```python
from build123d import *

# Parameters (mm, degrees)
BOSS_EXTRUDE1_DEPTH     = 5
SKETCH2_R               = 1.5
CUT_EXTRUDE1_DEPTH      = 5
CIRPATTERN1_COUNT       = 4
CIRPATTERN1_ANGLE       = 168
SKETCH9_W               = 120
SKETCH9_H               = 25
BOSS_EXTRUDE5_DEPTH     = 5
MIRROR3_COPY_1_SKETCH_R = 1.5
MIRROR3_COPY_1_DEPTH    = 5
MIRROR3_COPY_2_SKETCH_R = 1.5
MIRROR3_COPY_2_DEPTH    = 5
MIRROR3_COPY_3_SKETCH_R = 1.5
MIRROR3_COPY_3_DEPTH    = 5
SKETCH11_W              = 83.519878
SKETCH11_H              = 28.939674
CUT_EXTRUDE2_DEPTH      = 150
CHAMFER1_SIZE           = 1


with BuildPart() as part:
    # Sketch1 → Boss-Extrude1 (new body)
    with BuildSketch(Plane(origin=(0, 0, 0), x_dir=(1, 0, 0), z_dir=(0, 1, 0))):
        with BuildLine():
            Line((-60, 0), (-25.75, 0))
            Line((-25.75, 0), (25.75, 0))
            Line((25.75, 0), (60, 0))
            ThreePointArc((60, 0), (0, 60), (-60, 0))
        make_face()
    boss_extrude1 = extrude(amount=BOSS_EXTRUDE1_DEPTH)

    # Sketch2 → Cut-Extrude1 (cut)
    with BuildSketch(Plane(origin=(0, 5, 0), x_dir=(1, 0, 0), z_dir=(0, 1, 0))):
        with Locations((-54.772256, 5)):
            Circle(SKETCH2_R)
    cut_extrude1 = extrude(amount=-CUT_EXTRUDE1_DEPTH, mode=Mode.SUBTRACT)

    # CirPattern1: Cut-Extrude1 ×4 about axis
    cirpattern1_axis = Axis((0, 0, 0), (0, -1, 0))
    for i in range(1, CIRPATTERN1_COUNT):
        add(cut_extrude1.rotate(cirpattern1_axis, i * CIRPATTERN1_ANGLE / (CIRPATTERN1_COUNT - 1)), mode=Mode.SUBTRACT)

    # Sketch9 → Boss-Extrude5 (add)
    with BuildSketch(Plane.XY):
        with Locations((0, -7.5)):
            Rectangle(SKETCH9_W, SKETCH9_H)
    boss_extrude5 = extrude(amount=BOSS_EXTRUDE5_DEPTH)

    # Mirror3: Boss-Extrude1, Cut-Extrude1, Boss-Extrude5 across plane
    add(boss_extrude1.mirror(Plane.ZX.offset(5)))
    add(cut_extrude1.mirror(Plane.ZX.offset(5)), mode=Mode.SUBTRACT)
    add(boss_extrude5.mirror(Plane.ZX.offset(5)))

    # Mirror3 copy 1 sketch → Mirror3 copy 1 (cut)
    with BuildSketch(Plane(origin=(0, 5, 0), x_dir=(0.559193, 0, 0.829038), z_dir=(0, -1, 0))):
        with Locations((-54.772256, -5)):
            Circle(MIRROR3_COPY_1_SKETCH_R)
    extrude(amount=-MIRROR3_COPY_1_DEPTH, mode=Mode.SUBTRACT)

    # Mirror3 copy 2 sketch → Mirror3 copy 2 (cut)
    with BuildSketch(Plane(origin=(0, 5, 0), x_dir=(-0.374607, 0, 0.927184), z_dir=(0, -1, 0))):
        with Locations((-54.772256, -5)):
            Circle(MIRROR3_COPY_2_SKETCH_R)
    extrude(amount=-MIRROR3_COPY_2_DEPTH, mode=Mode.SUBTRACT)

    # Mirror3 copy 3 sketch → Mirror3 copy 3 (cut)
    with BuildSketch(Plane(origin=(0, 5, 0), x_dir=(-0.978148, 0, 0.207912), z_dir=(0, -1, 0))):
        with Locations((-54.772256, -5)):
            Circle(MIRROR3_COPY_3_SKETCH_R)
    extrude(amount=-MIRROR3_COPY_3_DEPTH, mode=Mode.SUBTRACT)

    # Sketch11 → Cut-Extrude2 (cut)
    with BuildSketch(Plane.ZY.offset(60)):
        with Locations((-36.759939, -9.469837)):
            Rectangle(SKETCH11_W, SKETCH11_H)
    extrude(amount=-CUT_EXTRUDE2_DEPTH, mode=Mode.SUBTRACT)

    # Chamfer1
    chamfer1_edges = [part.edges().sort_by_distance(p)[0] for p in [
        (0, 5, 5),
        (56.08213, 5, -6.808922),
        (-27.321858, 5, -49.447779),
        (60, 5, 2.5),
        (0, 5, -60),
        (25.715877, 5, -50.301694),
        (-56.272256, 5, -5),
        (-60, 5, 2.5),
    ]]
    chamfer(chamfer1_edges, length=CHAMFER1_SIZE)


solid = part.part
```
Source: CAD feature listing. Evaluate the final solid. Frame: model axes, mm. A direction names the side the tool comes from. Give positions to 0.01 mm unless a question says otherwise; leave off trailing zeros. Loops run counter-clockwise (first coordinate to the right, second up) from the corner with the lowest first, then second, coordinate; pieces in that order, holes last. Notation, with made-up numbers: (42.25, 10) -> (83.25, 10) arc R5 ccw to (83.25, 19) -> close; hole circle Ø10 at (-25, 63). An arc over 180 degrees is marked (long way). Use a Markdown table: item, result. Add a question column.
(1) Section query A-A (x = 0). Output: boundary loops of the cut face in (y, z), then the cut area to 3 significant figures.
(2) Ray query, line 1 (Z direction, x = -44.5, y = 27); line 2 (Y direction, x = 47, z = -24); line 3 (X direction, y = 7.5, z = -44). Return the intervals inside material, ascending.
(3) Access query for faces 5 (the face through (-1, 10, -24)), 6 (the face through (-1, 5, -21)). Directions: +Z, -Z, +X, -X, +Y, -Y. A direction counts if a zero-diameter tool reaches every point of the face in a straight line with its end or side. Return the directions, or none.
(4) Section query B-B (y = 24.25). Output: boundary loops of the cut face in (x, z), then the cut area to 3 significant figures.
(5) Pull-direction query (X, two-part tool) for faces 1 (the face through (25.654, 7.972, -50.325)), 2 (the face through (60, 18, 2)), 3 (the face through (1.319, 8.028, -59.985)), 4 (the face through (-1, 20, 0)); classes: +X half, -X half, draft (parallel to the pull), parting line (faces both ways), or undercut.
(6) First-contact query: pin 1 Ø4 at (x, z) = (-26.48, -48.2) entering from -Y; pin 2 Ø12 at (y, z) = (8.5, -41.5) entering from -X; pin 3 Ø2.5 at (x, z) = (25.15, -48.91) entering from -Y; pin 4 Ø6 at (x, y) = (-27.5, 18.5) entering from -Z. Flat tips, straight axial feed; report the tip coordinate or a pass-through.
Checked values:
| question | item | result |
|---|---|---|
| 1 | outline | (5, -59) -> (6, -60) -> (10, -60) -> (10, 0) -> (30, 0) -> (30, 5) -> (6, 5) -> (5, 4) -> close |
| 1 | area | 424 mm^2 |
| 2 | line 1 | 0 to 5 |
| 2 | line 2 | 5 to 10 |
| 2 | line 3 | -40.79 to 40.79 |
| 3 | face 5 | -Z, +X, -X, +Y |
| 3 | face 6 | +Z, -Z, +X, -X, -Y |
| 4 | outline | (-60, 0) -> (60, 0) -> (60, 5) -> (-60, 5) -> close |
| 4 | area | 600 mm^2 |
| 5 | face 1 | undercut |
| 5 | face 2 | +X half |
| 5 | face 3 | parting line |
| 5 | face 4 | draft |
| 6 | pin 1 | y = 5.49 |
| 6 | pin 2 | x = -48.37 |
| 6 | pin 3 | through |
| 6 | pin 4 | z = 0 |
